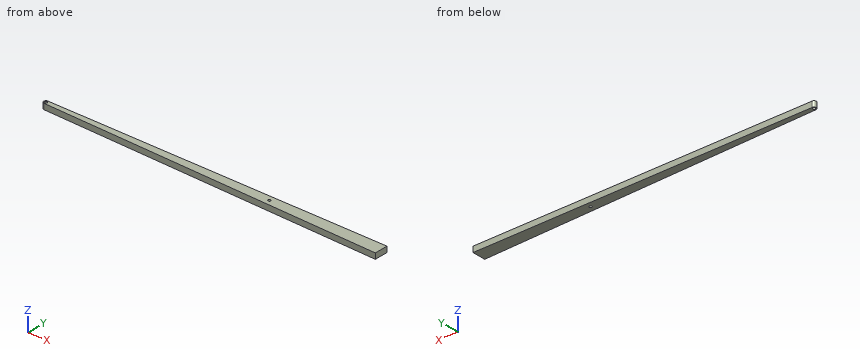
from build123d import *

# Parameters (mm, degrees)
F0_R     = 6
F1_DEPTH = 25


with BuildPart() as f1:
    # F0 (on Top) → F1 (new body)
    with BuildSketch(Plane.XY):
        with BuildLine():
            ThreePointArc((0, -10), (7.071068, -7.071068), (10, 0))
            ThreePointArc((10, 0), (7.071068, 7.071068), (0, 10))
            ThreePointArc((0, 10), (-10, 0), (0, -10))
        make_face()
        Circle(F0_R, mode=Mode.SUBTRACT)
        with BuildLine():
            ThreePointArc((0, 10), (7.071068, 7.071068), (10, 0))
            ThreePointArc((10, 0), (7.071068, -7.071068), (0, -10))
            Line((0, -10), (1500, -30))
            Line((1500, -30), (1500, 0))
            Line((1500, 0), (1500, 30))
            Line((1500, 30), (0, 10))
        make_face()
        with Locations((1000, 0)):
            Circle(F0_R, mode=Mode.SUBTRACT)
    extrude(amount=F1_DEPTH)


solid = f1.part
Geometry: final body of the model. Coordinates: model frame, mm. Round coordinates to 2 decimals unless told otherwise and drop trailing zeros. Order: outer loops, then holes, each group sorted by start corner. A loop starts at its lowest first (then second) coordinate and runs counter-clockwise, first axis right, second up. Notation, with made-up numbers: (-33, -23.75) -> (-24, -23.75) arc R29 cw to (-24, 15.25) -> close; hole circle Ø10 at (-38.5, 64.5). An arc over 180 degrees is marked (long way). Put each result on its own line as item: value. Start each with the question number.
Q1. Line query: probe 1 along X at (y, z) = (-2.5, 24); probe 2 along Y at (x, z) = (1000, 15.5); probe 3 along Y at (x, z) = (974, 15.75). Output: solid intervals per line, ascending.
Q2. First-contact query: pin 1 (15.5 mm diameter, centred on x = 0, y = 0, fed in from -Z); pin 2 (6 mm diameter, centred on x = 310.5, z = 9, fed in from -Y); pin 3 (11 mm diameter, centred on x = 1000, y = 0, fed in from -Z); pin 4 (10 mm diameter, centred on x = 155, z = 14, fed in from -Y). Flat tips, straight axial feed; report the tip coordinate or a pass-through.
Q3. Section B-B on x = 1398. Return the cut outline in (y, z), and give its area (3 significant figures).
Q4. Section C-C on x = 106. Return the cut outline in (y, z), and give its area (3 significant figures).
Q5. Section A-A on z = 11.25. Return the cut outline in (x, y), and give its area (3 significant figures).
Ans:
1. probe 1: x = -9.68 to -5.45, 5.45 to 994.55, 1005.45 to 1500
1. probe 2: y = -23.33 to -6, 6 to 23.33
1. probe 3: y = -22.99 to 22.99
2. pin 1: stops at z = 0
2. pin 2: stops at y = -14.18
2. pin 3: passes through
2. pin 4: stops at y = -12.13
3. outline: (-28.64, 0) -> (28.64, 0) -> (28.64, 25) -> (-28.64, 25) -> close
3. area: 1,430 mm2
4. outline: (-11.41, 0) -> (11.41, 0) -> (11.41, 25) -> (-11.41, 25) -> close
4. area: 571 mm2
5. outline: (0, -10) -> (1500, -30) -> (1500, 30) -> (0, 10) arc R10 ccw to start; hole circle Ø12 at (0, 0); hole circle Ø12 at (1000, 0)
5. area: 59,900 mm2
